The model under review builds one solid part; all positions refer to its coordinate system, in mm. A direction names the side the tool comes from. Coordinates: 2 decimals unless noted, no trailing zeros. Order: outer loops, then holes, each group sorted by start corner. A loop starts at its lowest first (then second) coordinate and runs counter-clockwise, first axis right, second up.
Autodesk Inventor part; units mm, degrees
ref_plane "YZ Plane" through (0, 0, 0) normal (1, 0, 0) x (0, 1, 0)
ref_plane "XZ Plane" through (0, 0, 0) normal (0, 1, 0) x (-1, 0, 0)
ref_plane "XY Plane" through (0, 0, 0) normal (0, 0, 1) x (1, 0, 0)
sketch "Skizze1" plane through (0, 0, 0) normal (0, 1, 0) x (-1, 0, 0)
  line L0 (-5, 0) -> (-62, 0)
  line L1 (-67, -5) -> (-67, -44)
  line L2 (-62, -49) -> (-5, -49)
  line L3 (0, -44) -> (0, -5)
  arc A0 (0, -5) -> (-5, 0) centre (-5, -5) ccw
  arc A1 (-62, 0) -> (-67, -5) centre (-62, -5) ccw
  arc A2 (-67, -44) -> (-62, -49) centre (-62, -44) ccw
  arc A3 (-5, -49) -> (0, -44) centre (-5, -44) ccw
  point P0 (0, 0)
  point P1 (-67, -49)
  point P2 (-67, 0)
  point P3 (0, -49)
  dimension "d0" = 67
  dimension "d1" = 49
  dimension "d2" = 5
extrude "Extrusion1" add sketch "Skizze1" along normal blind 2
sketch "Skizze2" plane through (0, 2, 0) normal (0, 1, 0) x (1, 0, 0)
  arc A0 (62, 0) -> (67, 5) centre (62, 5) ccw
  line L0 (67, 5) -> (67, 44)
  arc A1 (67, 44) -> (62, 49) centre (62, 44) ccw
  line L1 (62, 49) -> (5, 49)
  arc A2 (5, 49) -> (0, 44) centre (5, 44) ccw
  line L2 (0, 44) -> (0, 5)
  arc A3 (0, 5) -> (5, 0) centre (5, 5) ccw
  line L3 (5, 0) -> (62, 0)
  line L4 (6.9142, 5.5) -> (60.0858, 5.5)
  line L5 (60.0858, 5.5) -> (60.0858, 2)
  line L6 (60.0858, 2) -> (6.9142, 2)
  line L7 (6.9142, 2) -> (6.9142, 5.5)
  line L8 (61.5, 6.9142) -> (65, 6.9142)
  line L9 (65, 6.9142) -> (65, 42.0858)
  line L10 (65, 42.0858) -> (61.5, 42.0858)
  line L11 (61.5, 42.0858) -> (61.5, 6.9142)
  line L12 (60.0858, 47) -> (6.9142, 47)
  line L13 (6.9142, 47) -> (6.9142, 43.5)
  line L14 (6.9142, 43.5) -> (60.0858, 43.5)
  line L15 (60.0858, 43.5) -> (60.0858, 47)
  line L16 (2, 42.0858) -> (5.5, 42.0858)
  line L17 (5.5, 42.0858) -> (5.5, 6.9142)
  line L18 (5.5, 6.9142) -> (2, 6.9142)
  line L19 (2, 6.9142) -> (2, 42.0858)
  line L20 (33.5, 47) -> (33.5, 49) construction
  line L21 (65, 24.5) -> (67, 24.5) construction
  line L22 (62, 49) -> (5, 49) construction
  line L23 (33.5, 2) -> (33.5, 0) construction
  line L24 (5, 0) -> (62, 0) construction
  line L25 (2, 24.5) -> (0, 24.5) construction
  line L26 (0, 44) -> (0, 5) construction
  line L27 (5.5, 40.0858) -> (7, 40.0858)
  line L28 (7, 40.0858) -> (7, 42)
  line L29 (7, 42) -> (8.9142, 42)
  line L30 (8.9142, 42) -> (8.9142, 43.5)
  line L31 (61.5, 40.0858) -> (60, 40.0858)
  line L32 (60, 40.0858) -> (60, 42)
  line L33 (60, 42) -> (58.0858, 42)
  line L34 (58.0858, 42) -> (58.0858, 43.5)
  line L35 (61.5, 8.9142) -> (60, 8.9142)
  line L36 (60, 8.9142) -> (60, 7)
  line L37 (60, 7) -> (58.0858, 7)
  line L38 (58.0858, 7) -> (58.0858, 5.5)
  line L39 (8.9142, 5.5) -> (8.9142, 7)
  line L40 (8.9142, 7) -> (7, 7)
  line L41 (7, 7) -> (7, 8.9142)
  line L42 (7, 8.9142) -> (5.5, 8.9142)
  line L43 (2, 40.0858) -> (0, 40.0858)
  line L44 (65, 40.0858) -> (67, 40.0858)
  line L45 (65, 8.9142) -> (67, 8.9142)
  line L46 (58.0858, 2) -> (58.0858, 0)
  line L47 (8.9142, 2) -> (8.9142, 0)
  line L48 (2, 8.9142) -> (0, 8.9142)
  line L49 (8.9142, 47) -> (8.9142, 49)
  line L50 (58.0858, 47) -> (58.0858, 49)
  point P0 (0, 0)
  point P1 (58.0858, 0)
  point P2 (8.9142, 0)
  dimension "d5" = 3.5
  dimension "d6" = 2
  dimension "d7" = 35
  dimension "d9" = 2
  dimension "d10" = 2
  dimension "d11" = 2
extrude "Extrusion2" add sketch "Skizze2" along normal blind 2 contours L3 L47 L6 L46 | L45 L9 L44 L0 | L2 L43 L19 L48 | L50 L12 L49 L1
extrude "Extrusion3" add sketch "Skizze2" along normal blind 35 contours L3 L46 L6 L5 L4 L38 L37 L36 L35 L11 L8 L9 L45 L0 A0 | L3 A3 L2 L48 L19 L18 L17 L42 L41 L40 L39 L4 L7 L6 L47 | L44 L9 L10 L11 L31 L32 L33 L34 L14 L15 L12 L50 L1 A1 L0 | L2 A2 L1 L49 L12 L13 L14 L30 L29 L28 L27 L17 L16 L19 L43
equation "\"d10\" = d9"
properties part number "small_bottom"
(1) Wall thickness on line 1 (X direction, y = 25, z = -42.5); line 2 (Z direction, x = 6, y = 26); line 3 (Y direction, x = 12.5, z = -5): over which ranges is each line inside the solid? List them lowest first.
(2) Insertion check: pin 1 Ø2 at (x, z) = (19, -35.5) entering from +Y; pin 2 Ø2 at (x, y) = (0.5, 21) entering from -Z; pin 3 Ø1 at (x, z) = (26, -47.5) entering from +Y. Each pin has a flat end and moves straight along its axis. Give the tip position at first contact, or say it passes through.
(3) Tool access review of faces 4 (the face through (58.086, 20, -48)), 5 (the face through (63, 19, -6.914)), 6 (the face through (66, 20, -8.914)), 7 (the face through (62, 37, -45)): name each direction out of +Z, -Z, +X, -X, +Y, -Y from which nothing blocks a thin tool from reaching the whole face with its end or side.
(4) Consider section C-C (y = 25.5). Give the number of separate pieces and of enclosed holes in the cut face, then the cut area to 3 significant figures.
(5) Consider section A-A (z = -33.5). Give the boundary of the cut face in (x, y).
(6) Consider section B-B (x = 32.5). Give the boundary of the cut face in (y, z).
(7) The part is to be moulded in two halves that separate along Z. For faces 1 (the face through (33, 4, -48)), 2 (the face through (2, 18, -1)), 3 (the face through (1, 20, -40.086)), say which applies: +Z half, -Z half, draft (parallel to the pull), parting line (faces both ways), or undercut.
Findings:
1. line 1: x = 0 to 8.91, 58.09 to 67
1. line 2: z = -49 to -40.09, -8.91 to 0
1. line 3: y = 0 to 2
2. pin 1: stops at y = 2
2. pin 2: stops at z = -47.57
2. pin 3: stops at y = 4
3. face 4: +Z, -Z, +Y
3. face 5: +Y
3. face 6: +X, -X, +Y
3. face 7: +Z, -Z, +X, -X, +Y
4. separate pieces: 4
4. enclosed holes: 0
4. area: 226 mm2
5. outline: (0, 0) - (67, 0) - (67, 4) - (65, 4) - (65, 2) - (2, 2) - (2, 4) - (0, 4) - close
6. outline: (0, -49) - (4, -49) - (4, -47) - (2, -47) - (2, -2) - (4, -2) - (4, 0) - (0, 0) - close
7. face 1: draft
7. face 2: +Z half
7. face 3: undercut
